Autodesk Inventor part; units mm, degrees
ref_plane "YZ Plane" through (0, 0, 0) normal (1, 0, 0) x (0, 1, 0)
ref_plane "XZ Plane" through (0, 0, 0) normal (0, 1, 0) x (-1, 0, 0)
ref_plane "XY Plane" through (0, 0, 0) normal (0, 0, 1) x (1, 0, 0)
sketch "スケッチ1" plane through (0, 0, 0) normal (0, 0, 1) x (1, 0, 0)
  circle A0 centre (0, 0) radius 10.5 construction
  line L0 (0, 10.5) -> (-200, 10.5) construction
  line L1 (-200, 10.5) -> (-200, -10.5) construction
  line L2 (-200, -10.5) -> (0, -10.5) construction
  circle A1 centre (-195, 0) radius 1.55
  line L3 (-185, 2.5) -> (-70, 2.5) construction
  line L4 (-70, 2.5) -> (-70, -2.5) construction
  line L5 (-70, -2.5) -> (-185, -2.5) construction
  line L6 (-185, -2.5) -> (-185, 2.5) construction
  line L7 (-127.5, 2.5) -> (-127.5, -2.5) construction
  circle A2 centre (-60, 0) radius 1.55
  line L8 (-12, 21.3027) -> (-12, -27.3903) construction
  line L9 (-69.95, 2.55) -> (-185.05, 2.55) construction
  line L10 (-185.05, 2.55) -> (-185.05, -2.55) construction
  line L11 (-185.05, -2.55) -> (-69.95, -2.55) construction
  line L12 (-69.95, -2.55) -> (-69.95, 2.55) construction
  circle A3 centre (-184, 2.55) radius 1.05 construction
  line L13 (-185, 0) -> (-127.5, 0) construction
  line L14 (-185.05, 2.55) -> (-185.05, -2.55)
  arc A4 (-182.95, 2.55) -> (-185.05, 2.55) centre (-184, 2.55) ccw
  line L15 (-182.95, 2.55) -> (-72.05, 2.55)
  arc A5 (-69.95, 2.55) -> (-72.05, 2.55) centre (-71, 2.55) ccw
  line L16 (-69.95, 2.55) -> (-69.95, -2.55)
  arc A6 (-185.05, -2.55) -> (-182.95, -2.55) centre (-184, -2.55) ccw
  line L17 (-182.95, -2.55) -> (-72.05, -2.55)
  arc A7 (-72.05, -2.55) -> (-69.95, -2.55) centre (-71, -2.55) ccw
  circle A8 centre (0, 8.5) radius 1.35
  circle A9 centre (0, 0) radius 5.05
  circle A10 centre (-8.5, 0) radius 1.35
  circle A11 centre (0, -8.5) radius 1.35
  circle A12 centre (8.5, 0) radius 1.35
  line L18 (-200, 4.8006) -> (-200, -4.8006)
  line L19 (-200, 4.8006) -> (-60, 10.5)
  line L20 (-60, 10.5) -> (0, 10.5)
  line L21 (-200, -4.8006) -> (-60, -10.5)
  line L22 (-60, -10.5) -> (0, -10.5)
  arc A13 (0, -10.5) -> (0, 10.5) centre (0, 0) ccw
  circle A14 centre (-195, 0) radius 5 construction
  point P0 (-200, 0)
  dimension "d9" = 2.1
  dimension "d0" = 200
  dimension "d1" = 3.1
  dimension "d2" = 21
  dimension "d3" = 10
  dimension "d4" = 5
  dimension "d5" = 12
  dimension "d6" = 135
  dimension "d7" = 5
  dimension "d8" = 0.05
  dimension "d10" = 2.7
  dimension "d11" = 8.5
  dimension "d12" = 10.1
  dimension "d15" = 360
extrude "押し出し1" add sketch "スケッチ1" along normal blind 2
fillet "フィレット1" radius 2 2 edges at (-200, -4.8006, 1) (-200, 4.8006, 1)
equation "\"H_head\" = 28.5"
equation "\"H_leg\" = 199.5"
equation "\"足の面積\" = 12720.125"
equation "\"現在の面積\" = 11560"
equation "\"足_短辺\" = 68"
equation "\"円柱\" = 313.5"
equation "\"胴体中心から手先\" = 342"
equation "\"H_leg_1\" = 186.2"
equation "\"H_leg_MAX\" = 399"
equation "\"H_head_1\" = 26.6"
equation "\"H_head_MAX\" = 142.5"
properties part number "前腕_メインフレーム_1_1" material "GFRP"
Could you check a few things on this model? Use its own coordinates, in mm. Give positions to 0.01 mm unless a question says otherwise; leave off trailing zeros. Order: outer loops, then holes, each group sorted by start corner. A loop starts at its lowest first (then second) coordinate and runs counter-clockwise, first axis right, second up. Notation, with made-up numbers: (88.5, -31.75) -> (123.5, -31.75) arc R31 cw to (123.5, -5.75) -> close; hole circle Ø6 at (26, 85.25). An arc over 180 degrees is marked (long way). Return JSON: item names as keys, results as strings.
1. Imagine slicing it at A-A on z = 0.9. Give the number of separate pieces and of enclosed holes in the cut face, then the cut area to 3 significant figures.
Answer list:
{"separate pieces": "1", "enclosed holes": "8", "area": "2,860 mm2"}
2. Imagine slicing it at B-B on x = -101.5. List the corners of the cut face in (y, z) for me, then the cut area to 3 significant figures.
Answer list:
{"outline": "(-8.81, 0) -> (-2.55, 0) -> (-2.55, 2) -> (-8.81, 2) -> close; (2.55, 0) -> (8.81, 0) -> (8.81, 2) -> (2.55, 2) -> close", "area": "25.0 mm2"}
3. I need wall thicknesses on line 1 (Y direction, x = 0, z = 1.4); line 2 (X direction, y = -3, z = 0.75); line 3 (X direction, y = 4.25, z = 1.35). Which ranges of each line are inside material? Lowest first, please. Write a range as from..to.
Answer list:
{"line 1": "y = -10.5..-9.85, -7.15..-5.05, 5.05..7.15, 9.85..10.5", "line 2": "x = -200..-184.95, -183.05..-71.95, -70.05..-4.06, 4.06..10.06", "line 3": "x = -199.46..-2.73, 2.73..9.6"}
4. Thinking about a two-plate mould opening in Y: for faces 1 (the flat face through (-130.01, 7.65, 0.99)), 2 (the cylindrical face through (4.817, -1.517, 0.986)), 3 (the cylindrical face through (10.5, 0.2, 1)), 4 (the flat face through (-73, -5, 2)), which applies, pulls with the +Y half, pulls with the -Y half, needs draft (parallel to the pull), parting line crosses it, or undercut?
Answer list:
{"face 1": "pulls with the +Y half", "face 2": "undercut", "face 3": "parting line crosses it", "face 4": "needs draft"}
5. For pin 1 Ø5 at (x, y) = (-64.5, -6.5) entering from -Z; pin 2 Ø1 at (x, z) = (-134.5, 1) entering from +Y; pin 3 Ø0.6 at (y, z) = (-0.5, 1) entering from +X; pin 4 Ø0.6 at (x, z) = (-140.5, 1.5) entering from -Y, each with a flat end and sliding along its axis, tell me the tip position at first contact or that it passes through.
Answer list:
{"pin 1": "stops at z = 0", "pin 2": "stops at y = 7.49", "pin 3": "stops at x = 10.5", "pin 4": "stops at y = -7.24"}
